from build123d import *

# Parameters (mm, degrees)
F0_W     = 200
F0_H     = 100
F1_DEPTH = 15
F3_W     = 30.8789272606
F3_H     = 15
F4_DEPTH = 25
F5_R     = 10


with BuildPart() as f1:
    # F0 (on Top) → F1 (new body)
    with BuildSketch(Plane.XY):
        Rectangle(F0_W, F0_H)
    extrude(amount=F1_DEPTH)

    # F3 (on offset) → F4 (join)
    with BuildSketch(Plane.XZ.offset(25)):
        Polygon((10, 15), (85, 15), (85, 65), (10, 45), align=None)
        with Locations((54.5605363697, 37.5)):
            Rectangle(F3_W, F3_H, mode=Mode.SUBTRACT)
    extrude(amount=-F4_DEPTH)

    # F5
    f5_edges = [f1.edges().sort_by_distance(p)[0] for p in [
        (-100, 50, 7.5),
        (-100, -50, 7.5),
        (100, -50, 7.5),
        (100, 50, 7.5),
        (10, -12.5, 45),
        (85, -12.5, 65),
    ]]
    fillet(f5_edges, radius=F5_R)


solid = f1.part
For this review, take the finished solid that the model builds, in its own axes (mm). A direction names the side the tool comes from. Round coordinates to 2 decimals unless told otherwise and drop trailing zeros. Write each loop counter-clockwise with the first axis right and the second up, starting at its lowest first coordinate (ties: lowest second). Pieces come first, ordered by that corner, then holes. Notation, with made-up numbers: (-14.5, -26) - (13.5, -26) arc R3 ccw to (13.5, -22) - close; hole circle Ø1 at (17, 19). An arc over 180 degrees is marked (long way). Write item = value, one per line. Start each with the question number.
1. Draft analysis for pull direction X (two halves, no side actions). For faces 1 (the face through (-1, 1, 15)), 2 (the face through (54, -13, 45)), 3 (the face through (-100, -1, 7)), state which applies: released by +X, released by -X, zero draft, split by the parting line, or undercut.
2. Consider section D-D on z = 24. State the section outline as (x, y) points.
3. For pin 1 Ø23.5 at (x, z) = (30, 37.5) entering from +Y; pin 2 Ø5 at (x, z) = (68, 20.5) entering from -Y; pin 3 Ø3 at (y, z) = (-5, 33.5) entering from +X, all flat-tipped, find the tip position at first contact; note any pin that passes through.
4. Consider section B-B on x = 27. State the section outline as (y, z) points.
5. Consider section C-C on y = -28.5. State the section outline as (x, z) points.
6. For faces 4 (the face through (10, -13, 26)), 5 (the face through (47, 0, 28)), 6 (the face through (47, -25, 28)), 7 (the face through (54, -13, 30)), list the 3-axis set-ups (+Z, -Z, +X, -X, +Y, -Y) from which the entire face can be reached by the end or side of a thin tool; tool diameter is ignored.
7. Consider section A-A on z = 35. State the section outline as (x, y) points, plus the area to 3 significant figures.
8. Wall thickness on L1, parallel to X at y = -24, z = 27.5; L2, parallel to Z at x = -82, y = 22; L3, parallel to Z at x = 43.5, y = -18.5: over which ranges is each line inside the solid? List them lowest first.
Evaluation:
q1.face_1 = zero draft
q1.face_2 = undercut
q1.face_3 = released by -X
q2.outline = (10, -25) - (85, -25) - (85, 0) - (10, 0) - close
q3.pin_1 = 0
q3.pin_2 = -25
q3.pin_3 = 85
q4.outline = (-50, 0) - (50, 0) - (50, 15) - (0, 15) - (0, 49.53) - (-25, 49.53) - (-25, 15) - (-50, 15) - close
q5.outline = (-100, 0) - (100, 0) - (100, 15) - (-100, 15) - close
q6.face_4 = +Z, -X, +Y, -Y
q6.face_5 = +Z, +X, -X, +Y
q6.face_6 = +Z, +X, -X, -Y
q6.face_7 = +Y, -Y
q7.outline = (10, -25) - (39.12, -25) - (39.12, 0) - (10, 0) - close; (70, -25) - (85, -25) - (85, 0) - (70, 0) - close
q7.area = 1,100 mm2
q8.L1 = 10 to 85
q8.L2 = 0 to 15
q8.L3 = 0 to 30, 45 to 53.93
